```python
from build123d import *

# Parameters (mm, degrees)
EXTRUDE_1_DEPTH     = 250
SKETCH_7_R          = 8
CUT_EXTRUDE_2_DEPTH = 40


with BuildPart() as part:
    # 草图1 → 凸台-拉伸1 (new body)
    with BuildSketch(Plane.XY):
        with BuildLine():
            Line((0, 0), (54, 0))
            Line((54, 0), (54, 2.192931695))
            ThreePointArc((54, 2.192931695), (53.49587162, 3.698420478), (52.18680282, 4.596741564))
            Line((52.18680282, 4.596741564), (34.153085808, 9.749232139))
            ThreePointArc((34.153085808, 9.749232139), (31.534948207, 11.545874311), (30.526691448, 14.556851877))
            Line((30.526691448, 14.556851877), (30.526691448, 44.523721966))
            ThreePointArc((30.526691448, 44.523721966), (31.534948207, 47.534699532), (34.153085808, 49.331341705))
            Line((34.153085808, 49.331341705), (37.68680282, 50.340975136))
            ThreePointArc((37.68680282, 50.340975136), (38.99587162, 51.239296223), (39.5, 52.744785005))
            Line((39.5, 52.744785005), (39.5, 62.5))
            ThreePointArc((39.5, 62.5), (38.767766953, 64.267766953), (37, 65))
            Line((37, 65), (17, 65))
            ThreePointArc((17, 65), (15.232233047, 64.267766953), (14.5, 62.5))
            Line((14.5, 62.5), (14.5, 52.744785005))
            ThreePointArc((14.5, 52.744785005), (15.00412838, 51.239296223), (16.31319718, 50.340975136))
            Line((16.31319718, 50.340975136), (19.900297087, 49.316089449))
            ThreePointArc((19.900297087, 49.316089449), (22.518434689, 47.519447276), (23.526691448, 44.50846971))
            Line((23.526691448, 44.50846971), (23.526691448, 14.572104133))
            ThreePointArc((23.526691448, 14.572104133), (22.518434689, 11.561126567), (19.900297087, 9.764484395))
            Line((19.900297087, 9.764484395), (1.81319718, 4.596741564))
            ThreePointArc((1.81319718, 4.596741564), (0.50412838, 3.698420478), (0, 2.192931695))
            Line((0, 2.192931695), (0, 0))
        make_face()
    extrude(amount=EXTRUDE_1_DEPTH)

    # 草图7 → 切除-拉伸2 (cut)
    with BuildSketch(Plane(origin=(0, 0, 0), x_dir=(0, 0, -1), z_dir=(1, 0, 0))):
        with Locations(Location((-32, 30, 0), (0, 0, 90))):
            Circle(SKETCH_7_R)
        with Locations(Location((-102, 30, 0), (0, 0, 90))):
            Circle(SKETCH_7_R)
    extrude(amount=CUT_EXTRUDE_2_DEPTH, mode=Mode.SUBTRACT)


solid = part.part
```
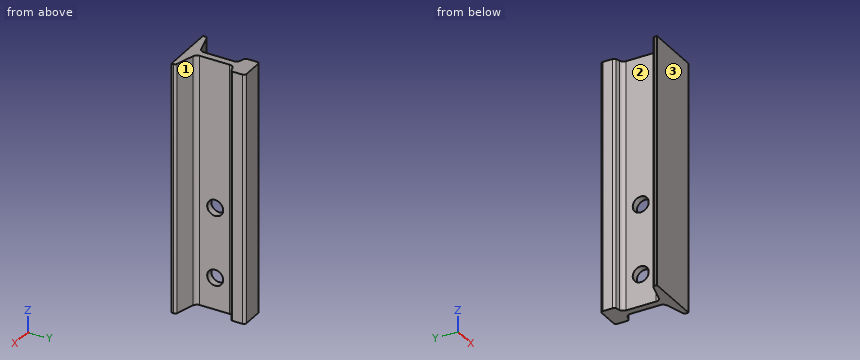
Input: part model. Units: mm. Frame: model coordinates. Face numbers are marked on the shaded views. Give positions to 0.01 mm unless a question says otherwise; leave off trailing zeros. Loops run counter-clockwise (first coordinate to the right, second up) from the corner with the lowest first, then second, coordinate; pieces in that order, holes last.
1) Section query B-B on y = 30. Return the cut outline in (x, z).
A:
outline: (23.53, 0) - (30.53, 0) - (30.53, 24) - (23.53, 24) - close; (23.53, 40) - (30.53, 40) - (30.53, 94) - (23.53, 94) - close; (23.53, 110) - (30.53, 110) - (30.53, 250) - (23.53, 250) - close
2) Section query C-C on x = 11. Return the cut outline in (y, z).
A:
outline: (0, 0) - (7.22, 0) - (7.22, 250) - (0, 250) - close
3) Section query A-A on z = 102. Return the cut outline in (x, y).
A:
outline: (0, 0) - (54, 0) - (54, 2.19) arc R2.5 ccw to (52.19, 4.6) - (34.15, 9.75) arc R5 cw to (30.53, 14.56) - (30.53, 22) - (23.53, 22) - (23.53, 14.57) arc R5 cw to (19.9, 9.76) - (1.81, 4.6) arc R2.5 ccw to (0, 2.19) - close; (14.5, 52.74) arc R2.5 ccw to (16.31, 50.34) - (19.9, 49.32) arc R5 cw to (23.53, 44.51) - (23.53, 38) - (30.53, 38) - (30.53, 44.52) arc R5 cw to (34.15, 49.33) - (37.69, 50.34) arc R2.5 ccw to (39.5, 52.74) - (39.5, 62.5) arc R2.5 ccw to (37, 65) - (17, 65) arc R2.5 ccw to (14.5, 62.5) - close
4) Line query: L1, parallel to Z at x = 27, y = 30; L2, parallel to Y at x = 25, z = 32; L3, parallel to X at y = 18, z = 29. Output: solid intervals per line, ascending.
A:
L1: z = 0 to 24, 40 to 94, 110 to 250
L2: y = 0 to 22, 38 to 65
L3: x = 23.53 to 30.53
5) Mould query, pull axis Y, two halves, no side actions, for the marked faces 1, 2 and 3. Classes: released by +Y, released by -Y, zero draft, split by the parting line, or undercut.
A:
face 1: undercut
face 2: undercut
face 3: released by -Y
6) Contact query for flat-ended pins moving along their axis: pin 1 (15 mm diameter, centred on y = 28.5, z = 175.5, fed in from -X); pin 2 (12 mm diameter, centred on y = 40, z = 26.5, fed in from -X); pin 3 (1.5 mm diameter, centred on x = 40.5, z = 62, fed in from +Y); pin 4 (5 mm diameter, centred on x = 23.5, y = 24, fed in from -Z). Output: stop coordinate, or through.
A:
pin 1: stops at x = 23.53
pin 2: stops at x = 23.3
pin 3: stops at y = 8.15
pin 4: stops at z = 0
